```python
from build123d import *

# Parameters (mm, degrees)
SKETCH_3_R      = 1.25
SKETCH_3_R_2    = 1.4
EXTRUDE_2_DEPTH = 10


with BuildPart() as part:
    # 草图3 → 凸台-拉伸2 (new body)
    with BuildSketch(Plane.XY):
        with BuildLine():
            Line((1203.23159256, 480.404853327), (1082.731592366, 480.404853327))
            Line((1082.731592366, 480.404853327), (1082.310142824, 480.826300075))
            ThreePointArc((1082.310142824, 480.826300075), (1082.163698991, 481.179854306), (1082.310145601, 481.533406638))
            Line((1082.310145601, 481.533406638), (1132.702661596, 531.925922701))
            ThreePointArc((1132.702661596, 531.925922701), (1135.946895085, 534.093650218), (1139.773729412, 534.854854894))
            Line((1139.773729412, 534.854854894), (1150.589455978, 534.854854894))
            ThreePointArc((1150.589455978, 534.854854894), (1154.416289827, 534.093650416), (1157.660523063, 531.925923433))
            Line((1157.660523063, 531.925923433), (1164.418316344, 525.168131543))
            Line((1164.418316344, 525.168131543), (1208.053038819, 481.533406638))
            ThreePointArc((1208.053038819, 481.533406638), (1208.199485429, 481.179853247), (1208.053038819, 480.826299856))
            Line((1208.053038819, 480.826299856), (1207.631592536, 480.404853327))
            Line((1207.631592536, 480.404853327), (1203.23159256, 480.404853327))
        make_face()
        with Locations((1113.18159221, 496.404853247)):
            Circle(SKETCH_3_R, mode=Mode.SUBTRACT)
        with Locations((1121.18159221, 496.404853247)):
            Circle(SKETCH_3_R, mode=Mode.SUBTRACT)
        with Locations((1129.18159221, 512.404853247)):
            Circle(SKETCH_3_R, mode=Mode.SUBTRACT)
        with Locations((1129.18159221, 504.404853247)):
            Circle(SKETCH_3_R, mode=Mode.SUBTRACT)
        with Locations((1129.18159221, 496.404853247)):
            Circle(SKETCH_3_R, mode=Mode.SUBTRACT)
        with Locations((1121.18159221, 504.404853247)):
            Circle(SKETCH_3_R, mode=Mode.SUBTRACT)
        with Locations((1169.18159221, 504.404853247)):
            Circle(SKETCH_3_R, mode=Mode.SUBTRACT)
        with Locations((1161.18159221, 496.404853247)):
            Circle(SKETCH_3_R, mode=Mode.SUBTRACT)
        with Locations((1161.18159221, 504.404853247)):
            Circle(SKETCH_3_R, mode=Mode.SUBTRACT)
        with Locations((1161.18159221, 512.404853247)):
            Circle(SKETCH_3_R, mode=Mode.SUBTRACT)
        with Locations((1169.18159221, 496.404853247)):
            Circle(SKETCH_3_R, mode=Mode.SUBTRACT)
        with Locations((1177.18159221, 496.404853247)):
            Circle(SKETCH_3_R, mode=Mode.SUBTRACT)
        with Locations((1137.68159221, 496.404853166)):
            Circle(SKETCH_3_R_2, mode=Mode.SUBTRACT)
        with Locations((1152.68159221, 496.404853166)):
            Circle(SKETCH_3_R_2, mode=Mode.SUBTRACT)
        with Locations((1137.68159221, 504.404852614)):
            Circle(SKETCH_3_R_2, mode=Mode.SUBTRACT)
        with Locations((1152.68159221, 504.404852614)):
            Circle(SKETCH_3_R_2, mode=Mode.SUBTRACT)
        with Locations((1137.68159221, 512.404853926)):
            Circle(SKETCH_3_R_2, mode=Mode.SUBTRACT)
        with Locations((1152.68159221, 512.404853926)):
            Circle(SKETCH_3_R_2, mode=Mode.SUBTRACT)
        with Locations((1137.68159221, 520.404851512)):
            Circle(SKETCH_3_R_2, mode=Mode.SUBTRACT)
        with Locations((1152.68159221, 520.404851512)):
            Circle(SKETCH_3_R_2, mode=Mode.SUBTRACT)
        with Locations((1137.68159221, 528.404852823)):
            Circle(SKETCH_3_R_2, mode=Mode.SUBTRACT)
        with Locations((1152.68159221, 528.404852823)):
            Circle(SKETCH_3_R_2, mode=Mode.SUBTRACT)
    extrude(amount=EXTRUDE_2_DEPTH)


solid = part.part
```
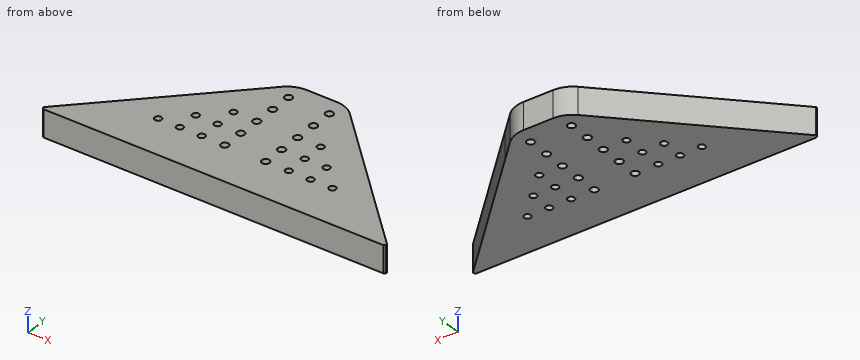
For this review, take the finished solid that the model builds, in its own axes (mm). Round coordinates to 2 decimals unless told otherwise and drop trailing zeros. Order: outer loops, then holes, each group sorted by start corner. A loop starts at its lowest first (then second) coordinate and runs counter-clockwise, first axis right, second up.
Q1. We need section A-A, the plane z = 2.75. State how many separate pieces and enclosed holes the cut face has, plus the area to 3 significant figures.
Findings below:
separate pieces: 1
enclosed holes: 22
area: 3,880 mm2
Q2. We need section C-C, the plane y = 509.5. Give the boundary of the cut face in (x, z).
Findings below:
outline: (1110.28, 0) - (1180.09, 0) - (1180.09, 10) - (1110.28, 10) - close
Q3. Insertion check: P1, Ø1, axis at x = 1157, z = 7.5, coming from the +Y side; P2, Ø2, axis at x = 1129.18, y = 496.4, coming from the +Z side; P3, Ø4.5, axis at x = 1152.68, y = 528.4, coming from the -Z side; P4, Ø2, axis at y = 499, z = 1, coming from the +X side. Each pin has a flat end and moves straight along its axis. Give the tip position at first contact, or say it passes through.
Findings below:
P1: stops at y = 532.92
P2: passes through
P3: stops at z = 0
P4: stops at x = 1191.59
Q4. We need section B-B, the plane x = 1156.5. Give the boundary of the cut face in (y, z), plus the area to 3 significant figures.
Findings below:
outline: (480.4, 0) - (532.92, 0) - (532.92, 10) - (480.4, 10) - close
area: 525 mm2
Q5. Wall thickness on line 1 (Y direction, x = 1139.5, z = 4); line 2 (X direction, y = 528.5, z = 8.5); line 3 (X direction, y = 500.5, z = 9.25): over which ranges is each line inside the solid? List them lowest first.
Findings below:
line 1: y = 480.4 to 534.85
line 2: x = 1129.28 to 1136.28, 1139.08 to 1151.28, 1154.08 to 1161.09
line 3: x = 1101.28 to 1189.09
